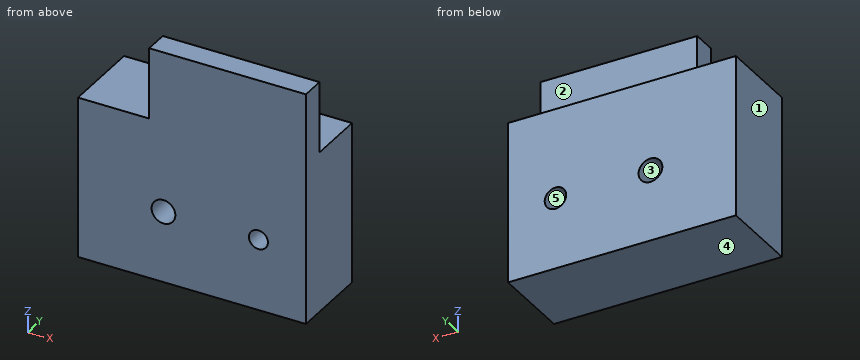
from build123d import *

# Parameters (mm, degrees)
SKETCH1_R           = 2.5
SKETCH1_R_2         = 2
BOSS_EXTRUDE1_DEPTH = 5
SKETCH2_W           = 48
SKETCH2_H           = 34
SKETCH2_R           = 2.5
SKETCH2_R_2         = 2.264702838
BOSS_EXTRUDE2_DEPTH = 12


with BuildPart() as part:
    # Sketch1 → Boss-Extrude1 (new body)
    with BuildSketch(Plane(origin=(0, 0, 0), x_dir=(1, 0, 0), z_dir=(0, 1, 0))):
        Polygon((15, 15), (15, 0), (48, 0), (48, 49), (0, 49), (0, 15), align=None)
        with Locations((18, 34)):
            Circle(SKETCH1_R, mode=Mode.SUBTRACT)
        with Locations((38, 34)):
            Circle(SKETCH1_R_2, mode=Mode.SUBTRACT)
    extrude(amount=BOSS_EXTRUDE1_DEPTH)

    # Sketch2 → Boss-Extrude2 (add)
    with BuildSketch(Plane(origin=(0, 5, 0), x_dir=(1, 0, 0), z_dir=(0, 1, 0))):
        with Locations((24, 32)):
            Rectangle(SKETCH2_W, SKETCH2_H)
        with Locations((18, 34)):
            Circle(SKETCH2_R, mode=Mode.SUBTRACT)
        with Locations((38, 34)):
            Circle(SKETCH2_R_2, mode=Mode.SUBTRACT)
    extrude(amount=BOSS_EXTRUDE2_DEPTH)


solid = part.part
Work out the finished part from the listing and answer in its coordinate system (mm). Face numbers are marked on the shaded views. A direction names the side the tool comes from. Coordinates: 2 decimals unless noted, no trailing zeros. Loops run counter-clockwise (first coordinate to the right, second up) from the corner with the lowest first, then second, coordinate; pieces in that order, holes last. Notation, with made-up numbers: M -13,-29.75 L 35,-29.75 A13 ccw 35,-9.75 Z; hole C 39.5,81.25 d3. An arc over 180 degrees is marked long. Answer in a Markdown table with one row per item. Add a question column.
1. Flat-ended cylindrical pins translate along their axes: P1, Ø7.5, axis at x = 38.5, z = -6, coming from the +Y side; P2, Ø1, axis at x = 9.5, y = 12.5, coming from the +Z side; P3, Ø10, axis at y = 4.5, z = -8.5, coming from the -X side; P4, Ø3, axis at x = 38, z = -34, coming from the +Y side. Find the tip coordinate at first contact, or state that the pin passes through.
2. Find section B-B, the plane z = -34. Write down the section's boundary in (x, y).
3. Find section D-D, the plane x = 18. Write down the section's boundary in (y, z), then the cut area to 3 significant figures.
4. Find section A-A, the plane x = 38. Write down the section's boundary in (y, z), then the cut area to 3 significant figures.
5. Find section C-C, the plane y = 2.25. Write down the section's boundary in (x, z).
6. Consider L1, parallel to X at y = 4.75, z = -34; L2, parallel to Z at x = 18, y = 7.5; L3, parallel to Z at x = 38, y = 2. Determine where each line is inside the solid, lowest interval first.
7. A tool of negligible diameter and unlimited length cuts with its end or side. For the marked faces 4 and 5, from which of +Z, -Z, +X, -X, +Y, -Y can it reach the whole face along a straight path? Write none if from no direction.
8. The mould has two halves that part along X. Classify the marked faces 1, 2 and 3: pulls with the +X half, pulls with the -X half, needs draft (parallel to the pull), parting line crosses it, or undercut.
Reported:
| question | item | result |
|---|---|---|
| 1 | P1 | stops at y = 5 |
| 1 | P2 | stops at z = -15 |
| 1 | P3 | stops at x = 15 |
| 1 | P4 | passes through |
| 2 | outline | M 0,0 L 15.5,0 L 15.5,17 L 0,17 Z; M 20.5,0 L 36,0 L 36,5 L 35.74,5 L 35.74,17 L 20.5,17 Z; M 40,0 L 48,0 L 48,17 L 40.26,17 L 40.26,5 L 40,5 Z |
| 3 | outline | M 0,-49 L 17,-49 L 17,-36.5 L 0,-36.5 Z; M 0,-31.5 L 17,-31.5 L 17,-15 L 5,-15 L 5,0 L 0,0 Z |
| 3 | area | 568 mm^2 |
| 4 | outline | M 0,-49 L 17,-49 L 17,-36.26 L 5,-36.26 L 5,-36 L 0,-36 Z; M 0,-32 L 5,-32 L 5,-31.74 L 17,-31.74 L 17,-15 L 5,-15 L 5,0 L 0,0 Z |
| 4 | area | 579 mm^2 |
| 5 | outline | M 0,-49 L 48,-49 L 48,0 L 15,0 L 15,-15 L 0,-15 Z; hole C 18,-34 d5; hole C 38,-34 d4 |
| 6 | L1 | x = 0 to 15.5, 20.5 to 36, 40 to 48 |
| 6 | L2 | z = -49 to -36.5, -31.5 to -15 |
| 6 | L3 | z = -49 to -36, -32 to 0 |
| 7 | face 4 | -Z, +X, -X, +Y, -Y |
| 7 | face 5 | +Y |
| 8 | face 1 | pulls with the -X half |
| 8 | face 2 | needs draft |
| 8 | face 3 | undercut |
